Can you work these out from the model? Positions are in its coordinate system, mm. A direction names the side the tool comes from. Round coordinates to 2 decimals unless told otherwise and drop trailing zeros. Loops run counter-clockwise (first coordinate to the right, second up) from the corner with the lowest first, then second, coordinate; pieces in that order, holes last. Notation, with made-up numbers: M 76,-37.5 L 105,-37.5 A13 cw 105,-31.5 Z; hole C -32,8 d9. An arc over 180 degrees is marked long. Return JSON: item names as keys, results as strings.
Autodesk Inventor part; units mm, degrees
ref_plane "YZ Plane" through (0, 0, 0) normal (1, 0, 0) x (0, 1, 0)
ref_plane "XZ Plane" through (0, 0, 0) normal (0, 1, 0) x (-1, 0, 0)
ref_plane "XY Plane" through (0, 0, 0) normal (0, 0, 1) x (1, 0, 0)
sketch "Sketch1" plane through (0, 0, 0) normal (0, 1, 0) x (-1, 0, 0)
  circle A0 centre (0, 0) radius 19.05
  dimension "d0" = 38.1
sketch "Sketch2" plane through (0, 0, 0) normal (1, 0, 0) x (0, 1, 0)
  line L0 (0, 0) -> (88.9, 0)
  arc A0 (114.8745, -25.9745) -> (88.9, 0) centre (88.9, -25.9745) ccw
  line L1 (114.8745, -25.9745) -> (114.8745, -203.7745)
  line L2 (0, -229.749) -> (88.9, -229.749)
  arc A1 (88.9, -229.749) -> (113.9345, -210.699) centre (88.9, -203.7745) ccw
  arc A2 (88.9, -229.749) -> (114.8745, -203.7745) centre (88.9, -203.7745) ccw
  dimension "d2" = 88.9
sweep "Sweep1" add profiles "Sketch1" path "Sketch2" path curves L0 A0 L1 A2 L2
sketch "Sketch3" plane through (0, 0, 0) normal (1, 0, 0) x (0, 1, 0)
  line L0 (95.8245, -25.9745) -> (133.9245, -25.9745)
  line L1 (133.9245, -25.9745) -> (133.9245, -203.7745)
  line L2 (133.9245, -25.9745) -> (133.9245, -203.7745)
  line L3 (133.9245, -114.8745) -> (95.8245, -114.8745)
  line L4 (95.8245, -25.9745) -> (95.8245, -203.7745)
  line L5 (89.4745, -89.4745) -> (140.2745, -89.4745)
  line L6 (140.2745, -89.4745) -> (140.2745, -140.2745)
  line L7 (140.2745, -140.2745) -> (89.4745, -140.2745)
  line L8 (89.4745, -140.2745) -> (89.4745, -89.4745)
  line L9 (89.4745, -89.4745) -> (140.2745, -140.2745) construction
  line L10 (140.2745, -89.4745) -> (89.4745, -140.2745) construction
  point P0 (0, 0)
  point P1 (114.8745, -114.8745)
  dimension "d8" = 50.8
  dimension "d9" = 50.8
extrude "Extrusion1" add sketch "Sketch3" along normal mid plane 50.8 contours L5 L1 L3 L4 | L4 L7 L8 L5 | L5 L6 L7 L1 | L3 L1 L7 L4
sketch "Sketch4" plane through (25.4, 0, 0) normal (1, 0, 0) x (0, 0, -1)
  line L0 (140.2745, 140.2745) -> (89.4745, 140.2745) construction
  line L1 (114.8745, 140.2745) -> (114.8745, 89.4745) construction
  line L2 (89.4745, 89.4745) -> (140.2745, 89.4745) construction
  line L3 (140.2745, 95.8245) -> (140.2745, 133.9245) construction
  line L4 (140.2745, 114.8745) -> (89.4745, 114.8745) construction
  line L5 (89.4745, 133.9245) -> (89.4745, 95.8245) construction
  circle A0 centre (114.8745, 114.8745) radius 6.35
  point P0 (0, 0)
  dimension "d23" = 12.7
extrude "Extrusion2" cut sketch "Sketch4" against normal through all
sketch "Sketch5" plane through (0, 0, 0) normal (1, 0, 0) x (0, 1, 0)
  line L0 (0, 0) -> (12.7, 0)
  line L1 (0, 0) -> (12.7, 0) construction
  line L2 (140.2745, -140.2745) -> (140.2745, -89.4745)
  line L3 (140.2745, -114.8745) -> (3.175, -114.8745)
  circle A0 centre (12.7, 0) radius 6.35
  circle A1 centre (12.7, -229.749) radius 6.35
  dimension "d16" = 12.7
  dimension "d21" = 12.7
  dimension "d22" = 12.7
extrude "Extrusion3" cut sketch "Sketch5" along normal through all both and the other way through all
properties part number "bogie (1)"
Q1. Thinking about a two-plate mould opening in Z: for faces 6 (the flat face through (0, 0, 0)), 7 (the cylindrical face through (0.356, 108.676, -113.498)), which applies, pulls with the +Z half, pulls with the -Z half, needs draft (parallel to the pull), parting line crosses it, or undercut?
Results:
{"face 6": "needs draft", "face 7": "undercut"}
Q2. Suppose I cut it at A-A, the plane y = 12.7. Please give me the cut outline in (x, z), plus the area to 3 significant figures.
Results:
{"outline": "M -17.96,-236.1 A19.05 ccw 17.96,-236.1 Z; M -17.96,-223.4 L 17.96,-223.4 A19.05 ccw Z; M -17.96,-6.35 A19.05 ccw 17.96,-6.35 Z; M -17.96,6.35 L 17.96,6.35 A19.05 ccw Z", "area": "1,330 mm2"}
Q3. On a 3-axis mill with a long thin cutter (end or side, diameter ignored), from which of +Z, -Z, +X, -X, +Y, -Y can I reach the whole of each face in a straight line? I mean faces 1 (the flat face through (-25.4, 109, -109)), 2 (the flat face through (0, 89.474, -115)), 3 (the cylindrical face through (0.267, 11.323, -235.948)), 4 (the cylindrical face through (-8.79, 43.83, -212.85)), 5 (the cylindrical face through (4.13, 96.278, -172.469)). Say none if no direction works.
Results:
{"face 1": "+Z, -Z, -X, +Y, -Y", "face 2": "+X, -X, -Y", "face 3": "+X, -X", "face 4": "-Y", "face 5": "none"}
Q4. Suppose I cut it at B-B, the plane x = -1. Please give me the cut outline in (y, z), plus the area to 3 significant figures.
Results:
{"outline": "M 0,-248.77 L 88.9,-248.77 A45 ccw 133.9,-203.77 L 133.9,-140.27 L 140.27,-140.27 L 140.27,-89.47 L 133.9,-89.47 L 133.9,-25.97 A45 ccw 88.9,19.02 L 0,19.02 L 0,-19.02 L 88.9,-19.02 A6.95 cw 95.85,-25.97 L 95.85,-89.47 L 89.47,-89.47 L 89.47,-140.27 L 95.85,-140.27 L 95.85,-203.77 A6.95 cw 88.9,-210.73 L 0,-210.73 Z; hole C 12.7,-229.75 d12.7; hole C 12.7,0 d12.7; hole C 114.87,-114.87 d12.7", "area": "16,900 mm2"}
Q5. Suppose I cut it at D-D, the plane z = -173.5. Please give me the cut outline in (x, y), plus the area to 3 significant figures.
Results:
{"outline": "C 0,114.87 d38.1", "area": "1,140 mm2"}
Q6. If I drill on line 1 along Z through (x, y) = (-0.5, 12.7); line 2 along Z through (x, y) = (-0.5, 51.5); line 3 along Z through (x, y) = (1.5, 12.7), over which ranges is the centre line in solid material (lowest first)?
Results:
{"line 1": "z = -248.79 to -236.1, -223.4 to -210.71, -19.04 to -6.35, 6.35 to 19.04", "line 2": "z = -248.79 to -210.71, -19.04 to 19.04", "line 3": "z = -248.74 to -236.1, -223.4 to -210.76, -18.99 to -6.35, 6.35 to 18.99"}
Q7. Suppose I cut it at C-C, the plane y = 56. Please give me the cut outline in (x, z).
Results:
{"outline": "C 0,-229.75 d38.1; C 0,0 d38.1"}
Q8. I'm going to push flat-ended pins straight in: pin 1 Ø1 at (x, z) = (12.5, -212.5) entering from -Y; pin 2 Ø5 at (x, y) = (9, 15.5) entering from +Z; pin 3 Ø16.5 at (y, z) = (114.87, -114.87) entering from +X; pin 4 Ø2 at (y, z) = (119, -215) entering from -X. Where does each tip first touch, or does it pass through?
Results:
{"pin 1": "stops at y = 95.63", "pin 2": "stops at z = 17.91", "pin 3": "stops at x = 25.4", "pin 4": "stops at x = -18.34"}
